from build123d import *

# Parameters (mm, degrees)
SKETCH1_W           = 36
SKETCH1_H           = 11.1
BOSS_EXTRUDE1_DEPTH = 1.5875
SKETCH2_W           = 5.4
SKETCH2_H           = 1.5875
CUT_EXTRUDE1_DEPTH  = 19.902980089


with BuildPart() as part:
    # Sketch1 → Boss-Extrude1 (new body)
    with BuildSketch(Plane(origin=(0, 0, 0), x_dir=(0, 0, -1), z_dir=(1, 0, 0))):
        Rectangle(SKETCH1_W, SKETCH1_H)
    extrude(amount=BOSS_EXTRUDE1_DEPTH)

    # Sketch2 → Cut-Extrude1 (cut, through all)
    with BuildSketch(Plane(origin=(1.5875, 0, 0), x_dir=(0, 0, -1), z_dir=(1, 0, 0))):
        with Locations((5.975, 4.75625)):
            Rectangle(SKETCH2_W, SKETCH2_H)
        with Locations((17.975, 4.75625)):
            Rectangle(SKETCH2_W, SKETCH2_H)
        with Locations((-6.025, 4.75625)):
            Rectangle(SKETCH2_W, SKETCH2_H)
        with Locations((-18.025, 4.75625)):
            Rectangle(SKETCH2_W, SKETCH2_H)
    cut_extrude1 = extrude(amount=-CUT_EXTRUDE1_DEPTH, mode=Mode.SUBTRACT)

    # Mirror1: Cut-Extrude1 across plane
    add(cut_extrude1.mirror(Plane.ZX), mode=Mode.SUBTRACT)


solid = part.part
For this review, take the finished solid that the model builds, in its own axes (mm). A direction names the side the tool comes from. Give positions to 0.01 mm unless a question says otherwise; leave off trailing zeros. Loops run counter-clockwise (first coordinate to the right, second up) from the corner with the lowest first, then second, coordinate; pieces in that order, holes last.
Item 1: For line 1 along Z through (x, y) = (1.15, -4) (3 decimals); line 2 along Y through (x, z) = (0.3, -4), list the stretches that pass through material, from the lowest coordinate up.
Item 2: Take a section at A-A, the plane y = 4.5. State the section outline as (x, z) points (1 decimal), and give its area (3 significant figures).
Item 3: Insertion check: pin 1 (0.5 mm diameter, centred on x = 0.5, y = 4.5, fed in from -Z) (3 decimals); pin 2 (0.8 mm diameter, centred on x = 1, z = 6, fed in from -Y). Each pin has a flat end and moves straight along its axis. Give the tip position at first contact, or say it passes through.
Item 4: Take a section at C-C, the plane z = 5.5. State the section outline as (x, y) points, and give its area (3 significant figures).
Item 5: Tool access review of faces 1 (the flat face through (1, -3.962, -17)), 2 (the flat face through (1, -5, 3.325)), 3 (the flat face through (1, 3.962, -17)), 4 (the flat face through (1, 3.962, -6)), 5 (the flat face through (1, 3.962, 17)): name each direction out of +Z, -Z, +X, -X, +Y, -Y from which nothing blocks a thin tool from reaching the whole face with its end or side.
Item 6: Draft analysis for pull direction Z (two halves, no side actions). For faces 6 (the flat face through (1, 5, 8.725)), 7 (the flat face through (1, -5.55, -12)), 8 (the flat face through (1, -5, -15.275)), state which applies: +Z half, -Z half, draft (parallel to the pull), parting line (faces both ways), or undercut.
Calculated:
1. line 1: z = -15.275 to -8.675, -3.275 to 3.325, 8.725 to 15.325
1. line 2: y = -3.96 to 3.96
2. outline: (0, -15.3) - (1.6, -15.3) - (1.6, -8.7) - (0, -8.7) - close; (0, -3.3) - (1.6, -3.3) - (1.6, 3.3) - (0, 3.3) - close; (0, 8.7) - (1.6, 8.7) - (1.6, 15.3) - (0, 15.3) - close
2. area: 31.4 mm2
3. pin 1: stops at z = -15.275
3. pin 2: stops at y = -3.96
4. outline: (0, -3.96) - (1.59, -3.96) - (1.59, 3.96) - (0, 3.96) - close
4. area: 12.6 mm2
5. face 1: -Z, +X, -X, -Y
5. face 2: +X, -X, -Y
5. face 3: -Z, +X, -X, +Y
5. face 4: +X, -X, +Y
5. face 5: +Z, +X, -X, +Y
6. face 6: undercut
6. face 7: draft
6. face 8: -Z half
